Geometry: see drawing. Coordinates: mm, zero at the bounding-box minimum. A direction names the side the tool comes from. Give positions to 0.01 mm unless a question says otherwise; leave off trailing zeros. Write each loop counter-clockwise with the first axis right and the second up, starting at its lowest first coordinate (ties: lowest second). Pieces come first, ordered by that corner, then holes. Notation, with made-up numbers: M -31.75,15.5 L 21.25,15.5 A14 cw 21.25,41.5 Z; hole C 14.25,32 d9. An arc over 180 degrees is marked long. Answer as a JSON object with one key per item and string values. Group by question number.
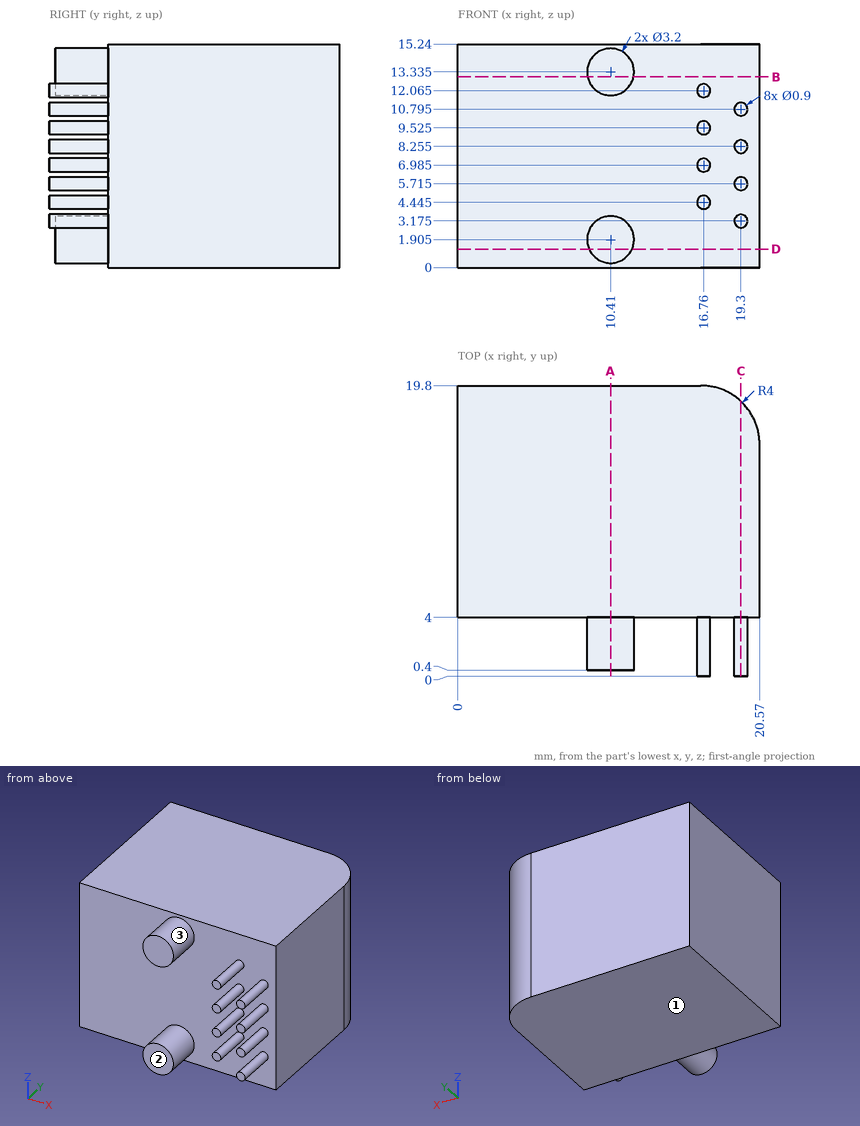
(1) Section D-D, the plane z = 1.25. Return loops of the section in (x, y), plus the area to 3 significant figures.
(2) Section B-B, the plane z = 13. Return loops of the section in (x, y).
(3) Section A-A, the plane x = 10.41. Return loops of the section in (y, z) (3 decimals).
(4) Ray query, L1, parallel to Y at x = 5, z = 10.75; L2, parallel to Y at x = 10, z = 1.5; L3, parallel to X at y = 16, z = 11.25 (3 decimals). Return the intervals inside material, ascending. Write a range as [from, to].
(5) Contact query for a flat-ended pin moving along its axis: pin 1 Ø7.5 at (x, z) = (11.5, 5.5) entering from -Y. Output: stop coordinate, or through.
(6) Section C-C, the plane x = 19.3. Return loops of the section in (y, z) (3 decimals).
(7) Access query for the marked faces 1, 2 and 3. Directions: +Z, -Z, +X, -X, +Y, -Y. A direction counts if a zero-diameter tool reaches every point of the face in a straight line with its end or side. Return the directions, or none.
Reported:
{
 "1": {"outline": "M 0,4 L 8.95,4 L 8.95,0.4 L 11.87,0.4 L 11.87,4 L 20.57,4 L 20.57,15.8 A4 ccw 16.57,19.8 L 0,19.8 Z", "area": "332 mm2"},
 "2": {"outline": "M 0,4 L 8.85,4 L 8.85,0.4 L 11.97,0.4 L 11.97,4 L 20.57,4 L 20.57,15.8 A4 ccw 16.57,19.8 L 0,19.8 Z"},
 "3": {"outline": "M 0.4,0.305 L 4,0.305 L 4,0 L 19.8,0 L 19.8,15.24 L 4,15.24 L 4,14.935 L 0.4,14.935 L 0.4,11.735 L 4,11.735 L 4,3.505 L 0.4,3.505 Z"},
 "4": {"L1": "y = [4, 19.8]", "L2": "y = [0.4, 19.8]", "L3": "x = [0, 20.565]"},
 "5": {"pin 1": "stops at y = 0.4"},
 "6": {"outline": "M 0,2.725 L 4,2.725 L 4,0 L 18.724,0 L 18.724,15.24 L 4,15.24 L 4,11.245 L 0,11.245 L 0,10.345 L 4,10.345 L 4,8.705 L 0,8.705 L 0,7.805 L 4,7.805 L 4,6.165 L 0,6.165 L 0,5.265 L 4,5.265 L 4,3.625 L 0,3.625 Z"},
 "7": {"face 1": "-Z, +X, -X, +Y, -Y", "face 2": "+Z, -Z, -X, -Y", "face 3": "-Y"}
}
